Check sheet for the modelled part. Datum: model origin and axes. Units: mm. Face numbers are marked on the shaded views. A direction names the side the tool comes from. Round coordinates to 2 decimals unless told otherwise and drop trailing zeros. Order: outer loops, then holes, each group sorted by start corner. A loop starts at its lowest first (then second) coordinate and runs counter-clockwise, first axis right, second up.
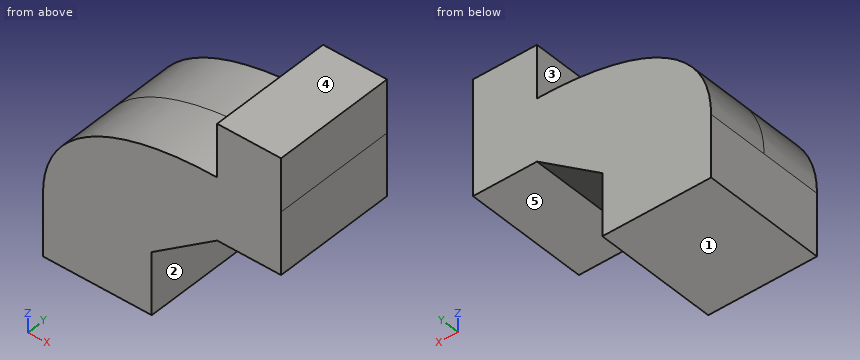
from build123d import *

# Parameters (mm, degrees)
F0_W     = 22.206857
F0_H     = 12.7
F0_W_2   = 13.062857
F1_DEPTH = 12.7
F2_DEPTH = 10.795


with BuildPart() as f1:
    # F0 (on Front) → F1 (new body, symmetric)
    with BuildSketch(Plane.XZ):
        with BuildLine():
            add(Edge.make_bspline(
                [(0, 12.7), (0, 29.538335), (18.433142, 35.12457), (35.559997, 34.834284)],
                knots=[0, 0, 0, 0, 41.886035, 41.886035, 41.886035, 41.886035], degree=3))
            Line((0, 12.7), (22.206857, 12.7))
            Line((22.206857, 12.7), (35.559997, 22.134284))
            Line((35.559997, 22.134284), (35.559997, 34.834284))
        make_face()
        with Locations((11.103428, 6.35)):
            Rectangle(F0_W, F0_H)
        with Locations((42.091425, 28.484284)):
            Rectangle(F0_W_2, F0_H)
    extrude(amount=F1_DEPTH, both=True)

    # F1_face (on face) → F2 (join)
    with BuildSketch(Plane(origin=(42.091425, 0, 34.834284), x_dir=(1, 0, 0), z_dir=(0, 0, 1))):
        Polygon((6.531428, -12.7), (6.531428, 12.7), (-6.531428, 12.7), (-6.531428, 0), (-6.531428, -12.7), align=None)
    extrude(amount=F2_DEPTH)


solid = f1.part
1) Gauge pin test, flat ends, axial feed: pin 1 (10 mm diameter, centred on x = 9.5, y = -5, fed in from +Z); pin 2 (4 mm diameter, centred on x = 39.5, y = 1, fed in from -Z); pin 3 (10 mm diameter, centred on y = 4, z = 4, fed in from +X); pin 4 (4 mm diameter, centred on x = 43.5, z = 19, fed in from -Y). Record the tip position at first contact, or that the pin passes through.
2) Sectioned sample at B-B on x = 36.5. Record the cut outline in (y, z), and give its area (3 significant figures).
3) Sectioned sample at A-A on z = 42. Record the cut outline in (x, y).
4) Set-up check for the marked faces 1 and 2: record each of +Z, -Z, +X, -X, +Y, -Y from which the full face is reachable in a straight line by a thin tool's end or side.
5) Scan lines: line 1 (X direction, y = 4.75, z = 42.5); line 2 (Z direction, x = 41.5, y = 1.5); line 3 (X direction, y = -6.25, z = 2). Record each from-to range of solid material in increasing order.
6) Draft check along Z on the marked faces 3, 4 and 5. Enter one of: pulls with the +Z half, pulls with the -Z half, needs draft (parallel to the pull), parting line crosses it, or undercut.
Values found:
1. pin 1: stops at z = 31.6
1. pin 2: stops at z = 22.13
1. pin 3: stops at x = 22.21
1. pin 4: passes through
2. outline: (-12.7, 22.13) - (12.7, 22.13) - (12.7, 45.63) - (-12.7, 45.63) - close
2. area: 597 mm2
3. outline: (35.56, -12.7) - (48.62, -12.7) - (48.62, 12.7) - (35.56, 12.7) - close
4. face 1: -Z, +X, -X, +Y, -Y
4. face 2: -Z, +X, +Y, -Y
5. line 1: x = 35.56 to 48.62
5. line 2: z = 22.13 to 45.63
5. line 3: x = 0 to 22.21
6. face 3: needs draft
6. face 4: pulls with the +Z half
6. face 5: pulls with the -Z half
